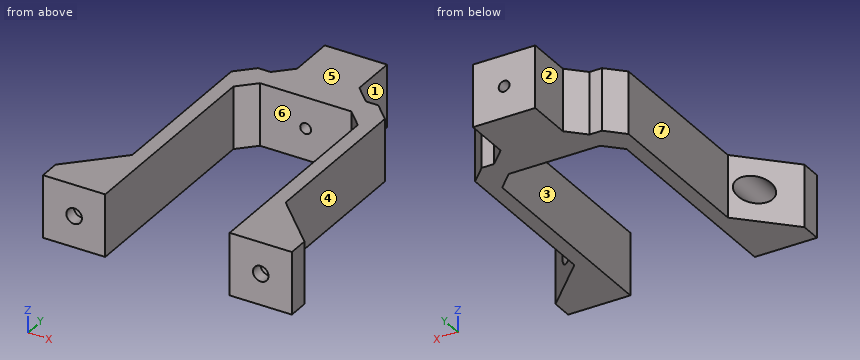
from build123d import *

# Parameters (mm, degrees)
SKETCH1_W             = 15
SKETCH1_H             = 15
SKETCH1_R             = 1.875
BOSS_EXTRUDE1_DEPTH   = 5
BOSS_EXTRUDE1_2_DEPTH = 5
SKETCH2_W             = 3.5
SKETCH2_H             = 15
BOSS_EXTRUDE2_DEPTH   = 50
SKETCH4_W             = 37
SKETCH4_H             = 15
BOSS_EXTRUDE3_DEPTH   = 5
SKETCH5_W             = 15
SKETCH5_H             = 15
BOSS_EXTRUDE4_DEPTH   = 15
SKETCH6_R             = 1.3
CUT_EXTRUDE1_DEPTH    = 82.124903698
CHAMFER1_SIZE         = 4
SKETCH7_R             = 3.25
CUT_EXTRUDE2_DEPTH    = 2
CHAMFER2_SIZE         = 11.5


with BuildPart() as part:
    # Sketch1 → Boss-Extrude1 (new body)
    with BuildSketch(Plane(origin=(0, 0, 0), x_dir=(1, 0, 0), z_dir=(0, 1, 0))):
        with Locations((-22.5, 0)):
            Rectangle(SKETCH1_W, SKETCH1_H)
        with Locations(Location((-22.5, 0, 0), (0, 0, 270))):
            Circle(SKETCH1_R, mode=Mode.SUBTRACT)
    extrude(amount=BOSS_EXTRUDE1_DEPTH)



with BuildPart() as body_2:
    # Sketch1 → Boss-Extrude1 2 (new body)
    with BuildSketch(Plane(origin=(0, 0, 0), x_dir=(1, 0, 0), z_dir=(0, 1, 0))):
        with Locations((22.5, 0)):
            Rectangle(SKETCH1_W, SKETCH1_H)
        with Locations(Location((22.5, 0, 0), (0, 0, 270))):
            Circle(SKETCH1_R, mode=Mode.SUBTRACT)
    extrude(amount=BOSS_EXTRUDE1_2_DEPTH)


with BuildPart() as part_1:
    add(part.part)

    add(body_2.part)  # Boss-Extrude2 merges body 2
    # Sketch2 → Boss-Extrude2 (add)
    with BuildSketch(Plane(origin=(0, 5, 0), x_dir=(1, 0, 0), z_dir=(0, 1, 0))):
        with Locations((-16.75, 0)):
            Rectangle(SKETCH2_W, SKETCH2_H)
        with Locations((16.75, 0)):
            Rectangle(SKETCH2_W, SKETCH2_H)
    extrude(amount=BOSS_EXTRUDE2_DEPTH)

    # Sketch4 → Boss-Extrude3 (add)
    with BuildSketch(Plane(origin=(0, 55, 0), x_dir=(1, 0, 0), z_dir=(0, 1, 0))):
        Rectangle(SKETCH4_W, SKETCH4_H)
    extrude(amount=BOSS_EXTRUDE3_DEPTH)

    # Sketch5 → Boss-Extrude4 (add)
    with BuildSketch(Plane(origin=(0, 60, 0), x_dir=(1, 0, 0), z_dir=(0, 1, 0))):
        Rectangle(SKETCH5_W, SKETCH5_H)
    extrude(amount=BOSS_EXTRUDE4_DEPTH)

    # Sketch6 → Cut-Extrude1 (cut, through all)
    with BuildSketch(Plane(origin=(0, 75, 0), x_dir=(1, 0, 0), z_dir=(0, 1, 0))):
        with Locations(Location((0, 0, 0), (0, 0, 270))):
            Circle(SKETCH6_R)
    extrude(amount=-CUT_EXTRUDE1_DEPTH, mode=Mode.SUBTRACT)

    # Chamfer1
    chamfer1_edges = [part_1.edges().sort_by_distance(p)[0] for p in [
        (-15, 55, 0),
        (-18.5, 60, 0),
        (18.5, 60, 0),
        (15, 55, 0),
        (7.5, 60, 0),
        (-7.5, 60, 0),
    ]]
    chamfer(chamfer1_edges, length=CHAMFER1_SIZE)

    # Sketch7 → Cut-Extrude2 (cut)
    with BuildSketch(Plane(origin=(0, 5, 0), x_dir=(1, 0, 0), z_dir=(0, 1, 0))):
        with Locations(Location((-22.5, 0, 0), (0, 0, 270))):
            Circle(SKETCH7_R)
        with Locations(Location((22.5, 0, 0), (0, 0, 270))):
            Circle(SKETCH7_R)
    extrude(amount=-CUT_EXTRUDE2_DEPTH, mode=Mode.SUBTRACT)

    # Chamfer2
    # the kernel refuses this chamfer: 11.5 mm, written as the material it adds along each edge
    with BuildSketch(Plane(origin=(18.5, 5, 7.5), x_dir=(0.9996219169112968, -0.02749587661058638, 0), z_dir=(0, 0, -1))) as chamfer2_piece_1_section:
        Polygon((CHAMFER2_SIZE * 0.999621916911, -CHAMFER2_SIZE * 0.0274958766106), (-CHAMFER2_SIZE * 0.0274958766106, -CHAMFER2_SIZE * 0.999621916911), (0, 0), align=None)
    chamfer2_piece_1 = extrude(amount=15, mode=Mode.PRIVATE)
    chamfer2_piece_1 = split(chamfer2_piece_1, bisect_by=Plane(origin=(30, 6.904321088, -5), z_dir=(-1, 0, 0)), keep=Keep.TOP, mode=Mode.PRIVATE)
    chamfer2_piece_1 = chamfer2_piece_1 - Plane(origin=(22.5, 6.904321088, 0), x_dir=(0, 0, 1), z_dir=(0, 1, 0)) * Cylinder(3.25, 76, mode=Mode.PRIVATE)
    add(chamfer2_piece_1)
    with BuildSketch(Plane(origin=(-18.5, 5, -7.5), x_dir=(-0.9996219169112968, -0.02749587661058638, 0), z_dir=(0, 0, 1))) as chamfer2_piece_2_section:
        Polygon((CHAMFER2_SIZE * 0.999621916911, -CHAMFER2_SIZE * 0.0274958766106), (-CHAMFER2_SIZE * 0.0274958766106, -CHAMFER2_SIZE * 0.999621916911), (0, 0), align=None)
    chamfer2_piece_2 = extrude(amount=15, mode=Mode.PRIVATE)
    chamfer2_piece_2 = split(chamfer2_piece_2, bisect_by=Plane(origin=(-30, 6.90432124, 5), z_dir=(1, 0, 0)), keep=Keep.TOP, mode=Mode.PRIVATE)
    chamfer2_piece_2 = chamfer2_piece_2 - Plane(origin=(-22.5, 6.90432124, 0), x_dir=(0, 0, 1), z_dir=(0, 1, 0)) * Cylinder(3.25, 76, mode=Mode.PRIVATE)
    add(chamfer2_piece_2)


solid = part_1.part
Design review of the part built by this model. Coordinates are the model's own, in mm. Face numbers are marked on the shaded views. A direction names the side the tool comes from. Give positions to 0.01 mm unless a question says otherwise; leave off trailing zeros. Loops run counter-clockwise (first coordinate to the right, second up) from the corner with the lowest first, then second, coordinate; pieces in that order, holes last. Notation, with made-up numbers: M -2.5,-21.5 L 55.5,-21.5 A16 cw 55.5,-11.5 Z; hole C -1,39 d4. An arc over 180 degrees is marked long. Answer as a JSON object with one key per item and string values.
Item 1: Mouldability with a two-part tool opening along X and no side actions: class the marked faces 4, 5, 6 and 7 as pulls with the +X half, pulls with the -X half, needs draft (parallel to the pull), parting line crosses it, or undercut.
Output values:
{"face 4": "pulls with the +X half", "face 5": "needs draft", "face 6": "undercut", "face 7": "pulls with the -X half"}
Item 2: For P1, Ø2, axis at x = 24, z = 0, coming from the +Y side; P2, Ø2.5, axis at x = -12.5, z = 0, coming from the +Y side; P3, Ø0.9, axis at x = 12.5, z = 3.5, coming from the +Y side, all flat-tipped, find the tip position at first contact; note any pin that passes through.
Output values:
{"P1": "stops at y = 3", "P2": "stops at y = 60.25", "P3": "stops at y = 60"}
Item 3: We need section D-D (y = 68.5). State the section outline as (x, z) points, and give its area (3 significant figures).
Output values:
{"outline": "M -7.5,-7.5 L 7.5,-7.5 L 7.5,7.5 L -7.5,7.5 Z; hole C 0,0 d2.6", "area": "220 mm2"}
Item 4: Wall thickness on line 1 along X through (y, z) = (1.95, 0) (3 decimals); line 2 along X through (y, z) = (21, 4.25); line 3 along Z through (x, y) = (-22.5, 2.2) (3 decimals): over which ranges is each line inside the solid? List them lowest first.
Output values:
{"line 1": "x = -30 to -24.375, -20.625 to -15, 15 to 20.625, 24.375 to 30", "line 2": "x = -18.5 to -15, 15 to 18.5", "line 3": "z = -7.5 to -1.875, 1.875 to 7.5"}
Item 5: Machinability: for the marked faces 1, 2 and 3, which of the approach directions +Z, -Z, +X, -X, +Y, -Y give a long, thin tool a straight path to every point of the face, cutting with its end or side? Answer none if there is none.
Output values:
{"face 1": "+Z, -Z, +X, +Y", "face 2": "+Z, -Z, -X, +Y", "face 3": "+Z, -Z, -Y"}
Item 6: We need section A-A (y = 36). State the section outline as (x, z) points, and give its area (3 significant figures).
Output values:
{"outline": "M -18.5,-7.5 L -15,-7.5 L -15,7.5 L -18.5,7.5 Z; M 15,-7.5 L 18.5,-7.5 L 18.5,7.5 L 15,7.5 Z", "area": "105 mm2"}
Item 7: We need section B-B (x = 0). State the section outline as (y, z) points, and give its area (3 significant figures).
Output values:
{"outline": "M 55,-7.5 L 75,-7.5 L 75,-1.3 L 55,-1.3 Z; M 55,1.3 L 75,1.3 L 75,7.5 L 55,7.5 Z", "area": "248 mm2"}
Item 8: We need section C-C (z = -5.5). State the section outline as (x, y) points.
Output values:
{"outline": "M -30,0 L -15,0 L -15,51 L -11,55 L 11,55 L 15,51 L 15,0 L 30,0 L 30,5 L 18.5,16.5 L 18.5,56 L 14.5,60 L 11.5,60 L 7.5,64 L 7.5,75 L -7.5,75 L -7.5,64 L -11.5,60 L -14.5,60 L -18.5,56 L -18.5,16.5 L -30,5 Z"}
